from build123d import *

# Parameters (mm, degrees)
F0_R      = 6.35
F1_DEPTH  = 19.05
F3_D      = 5.08
F8_D      = 3.048
F8_DEPTH  = 2.54
F8_TIP    = 0.9157115834
F9_D      = 3.048
F9_DEPTH  = 2.54
F9_TIP    = 0.9157115834
F11_D     = 11.938
F11_DEPTH = 12.7
F11_TIP   = 3.586537035


# Not quite as in the source:
# - the program builds the solid bodies; features that only make, move or delete a surface that nothing else refers to are left out


with BuildPart() as f1:
    # F0 (on Top) → F1 (new body)
    with BuildSketch(Plane.XY):
        Circle(F0_R)
    extrude(amount=F1_DEPTH)

    # F3 (through all)
    with Locations(Plane(origin=(0, 0, 0), x_dir=(1, 0, 0), z_dir=(0, 0, -1))):
        with Locations((0, 0)):
            Hole(F3_D / 2)

    # F8
    with Locations(Plane.XY.offset(19.05)):
        with Locations((0, 4.4337138534)):
            Hole(F8_D / 2, depth=F8_DEPTH)
            with Locations((0, 0, -(F8_DEPTH + F8_TIP / 2))):  # 118° drill point
                Cone(0, F8_D / 2, F8_TIP, mode=Mode.SUBTRACT)

    # F9
    with Locations(Plane.XY.offset(19.05)):
        with Locations((0, -4.445)):
            Hole(F9_D / 2, depth=F9_DEPTH)
            with Locations((0, 0, -(F9_DEPTH + F9_TIP / 2))):  # 118° drill point
                Cone(0, F9_D / 2, F9_TIP, mode=Mode.SUBTRACT)

    # F11
    with Locations(Plane(origin=(0, 0, 0), x_dir=(1, 0, 0), z_dir=(0, 0, -1))):
        with Locations((0, 0)):
            Hole(F11_D / 2, depth=F11_DEPTH)
            with Locations((0, 0, -(F11_DEPTH + F11_TIP / 2))):  # 118° drill point
                Cone(0, F11_D / 2, F11_TIP, mode=Mode.SUBTRACT)


solid = f1.part
Model file for the job. Use its own axes, mm. A direction names the side the tool comes from. Coordinates: 2 decimals unless noted, no trailing zeros. Order: outer loops, then holes, each group sorted by start corner. A loop starts at its lowest first (then second) coordinate and runs counter-clockwise, first axis right, second up. Notation, with made-up numbers: (63, 33) -> (71, 33) arc R22 cw to (71, 50) -> close; hole circle Ø5 at (88, 82.5). An arc over 180 degrees is marked (long way). Return JSON: item names as keys, results as strings. Group by question number.
Item 1: Tool access for faces 1 (the conical face through (2.63, -0.83, 14.63)), 2 (the cylindrical face through (0.33, -5.933, 17.762)): list every direction of +Z, -Z, +X, -X, +Y, -Y with a clear straight run to the whole face (end or side of a thin tool).
Item 2: Pull direction Y, two halves, no side cores. Call faces 3 (the flat face through (-0.1, -2.7, 19.05)), 4 (the cylindrical face through (-1.38, -6.2, 9.39)), 5 (the cylindrical face through (1.294, 5.827, 6.439)): pulls with the +Y half, pulls with the -Y half, needs draft (parallel to the pull), parting line crosses it, or undercut.
Item 3: Flat gauge pins, fed straight in: P1, Ø3, axis at y = -4, z = 6, coming from the -X side; P2, Ø6.5, axis at x = 0, y = 0, coming from the -Z side; P3, Ø2.5, axis at x = 0, y = 4.43, coming from the -Z side. Where does each tip first touch, or does it go through?
Item 4: Wall check: line 1 along Y through (x, z) = (0, 16.6); line 2 along X through (y, z) = (-5.25, 12.25); line 3 along Y through (x, z) = (-1, 1). Give the ranges that are in metal, low to high. Write a range as [from, to].
Item 5: Saw through at A-A on y = 0. Write the cut outline in (x, z), then the cut area to 3 significant figures.
Item 6: Saw through at B-B on z = 6.25. Write the cut outline in (x, y), then the cut area to 3 significant figures.
Values found:
{
 "1": {"face 1": "-Z", "face 2": "+Z"},
 "2": {"face 3": "needs draft", "face 4": "parting line crosses it", "face 5": "undercut"},
 "3": {"P1": "stops at x = -5.84", "P2": "stops at z = 14.33", "P3": "stops at z = 12.87"},
 "4": {"line 1": "y = [-6.35, -5.97], [-2.92, -2.54], [2.54, 2.91], [5.96, 6.35]", "line 2": "x = [-3.57, -2.84], [2.84, 3.57]", "line 3": "y = [-6.27, -5.88], [5.88, 6.27]"},
 "5": {"outline": "(-6.35, 0) -> (-5.97, 0) -> (-5.97, 12.7) -> (-2.54, 14.76) -> (-2.54, 19.05) -> (-6.35, 19.05) -> close; (2.54, 14.76) -> (5.97, 12.7) -> (5.97, 0) -> (6.35, 0) -> (6.35, 19.05) -> (2.54, 19.05) -> close", "area": "51.0 mm2"},
 "6": {"outline": "circle Ø12.7 at (0, 0); hole circle Ø11.94 at (0, 0)", "area": "14.7 mm2"}
}
